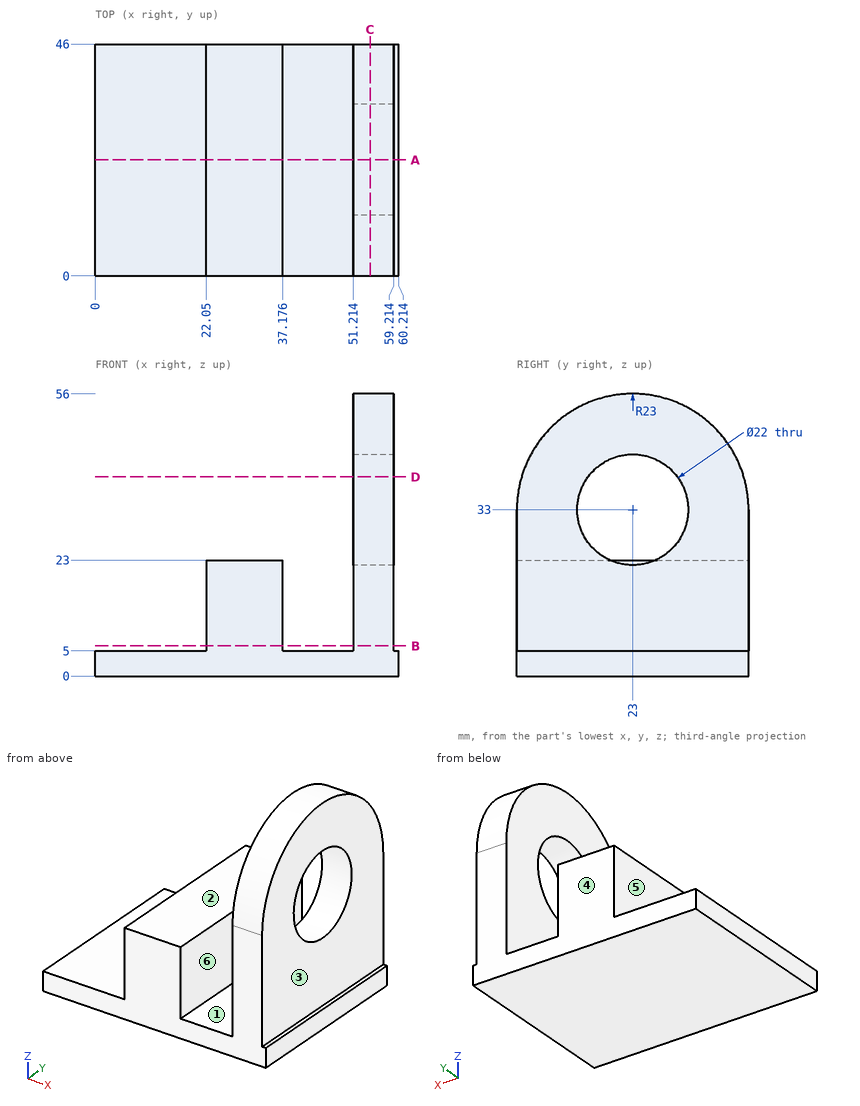
Study the drawing (mm; zero at the part's minimum x, y, z) and answer. A direction names the side the tool comes from. Coordinates: 2 decimals unless noted, no trailing zeros. Write each loop counter-clockwise with the first axis right and the second up, starting at its lowest first coordinate (ties: lowest second). Pieces come first, ordered by that corner, then holes. Notation, with made-up numbers: (10.5, -0.75) -> (42.5, -0.75) arc R16 cw to (42.5, 10.25) -> close; hole circle Ø10 at (66, -28). An arc over 180 degrees is marked (long way). Write each question's results on one line, items separated by ' | '. Start each with the question number.
1) A cutting plane is placed at C-C (x = 54.5). Determine the outline of the cut face in (y, z), then the cut area to 3 significant figures.
2) A tool of negligible diameter and unlimited length cuts with its end or side. For the marked faces 4, 5 and 6, from which of +Z, -Z, +X, -X, +Y, -Y can it reach the whole face along a straight path? Write none if from no direction.
3) Straight lines are drawn through the part: probe 1 along X at (y, z) = (19, 8); probe 2 along Y at (x, z) = (56, 33); probe 3 along Z at (x, y) = (45, 17.5). For each, find the intervals that lie inside material, in ascending order.
4) A cutting plane is placed at A-A (y = 23). Determine the outline of the cut face in (x, z).
5) A cutting plane is placed at B-B (z = 6). Determine the outline of the cut face in (x, y).
6) A cutting plane is placed at D-D (z = 39.5). Determine the outline of the cut face in (x, y), then the cut area to 3 significant figures.
7) For a pull along X with two mould halves and no side action, classify the marked faces 1, 2 and 3 as +X half, -X half, draft (parallel to the pull), parting line (faces both ways), or undercut.
8) Flat-ended cylindrical pins translate along their axes: pin 1 Ø6 at (y, z) = (9.5, 13) entering from +X; pin 2 Ø5 at (x, y) = (37.5, 28.5) entering from +Z; pin 3 Ø11 at (x, y) = (14.5, 34) entering from +Z. Find the tip coordinate at first contact, or state that the pin passes through.
Values follow:
1) outline: (0, 0) -> (46, 0) -> (46, 33) arc R23 ccw to (0, 33) -> close; hole circle Ø22 at (23, 33) | area: 1,970 mm²
2) face 4: +Z, -Z, +X, -X, +Y | face 5: +Z, -X, +Y, -Y | face 6: +Z, +Y, -Y
3) probe 1: 22.05 to 37.18, 51.21 to 59.21 | probe 2: 0 to 12, 34 to 46 | probe 3: 0 to 5
4) outline: (0, 0) -> (60.21, 0) -> (60.21, 5) -> (59.21, 5) -> (59.21, 22) -> (51.21, 22) -> (51.21, 5) -> (37.18, 5) -> (37.18, 23) -> (22.05, 23) -> (22.05, 5) -> (0, 5) -> close; (51.21, 44) -> (59.21, 44) -> (59.21, 56) -> (51.21, 56) -> close
5) outline: (22.05, 0) -> (37.18, 0) -> (37.18, 46) -> (22.05, 46) -> close; (51.21, 0) -> (59.21, 0) -> (59.21, 46) -> (51.21, 46) -> close
6) outline: (51.21, 0.94) -> (59.21, 0.94) -> (59.21, 14.13) -> (51.21, 14.13) -> close; (51.21, 31.87) -> (59.21, 31.87) -> (59.21, 45.06) -> (51.21, 45.06) -> close | area: 211 mm²
7) face 1: undercut | face 2: draft | face 3: +X half
8) pin 1: x = 59.21 | pin 2: z = 23 | pin 3: z = 5
